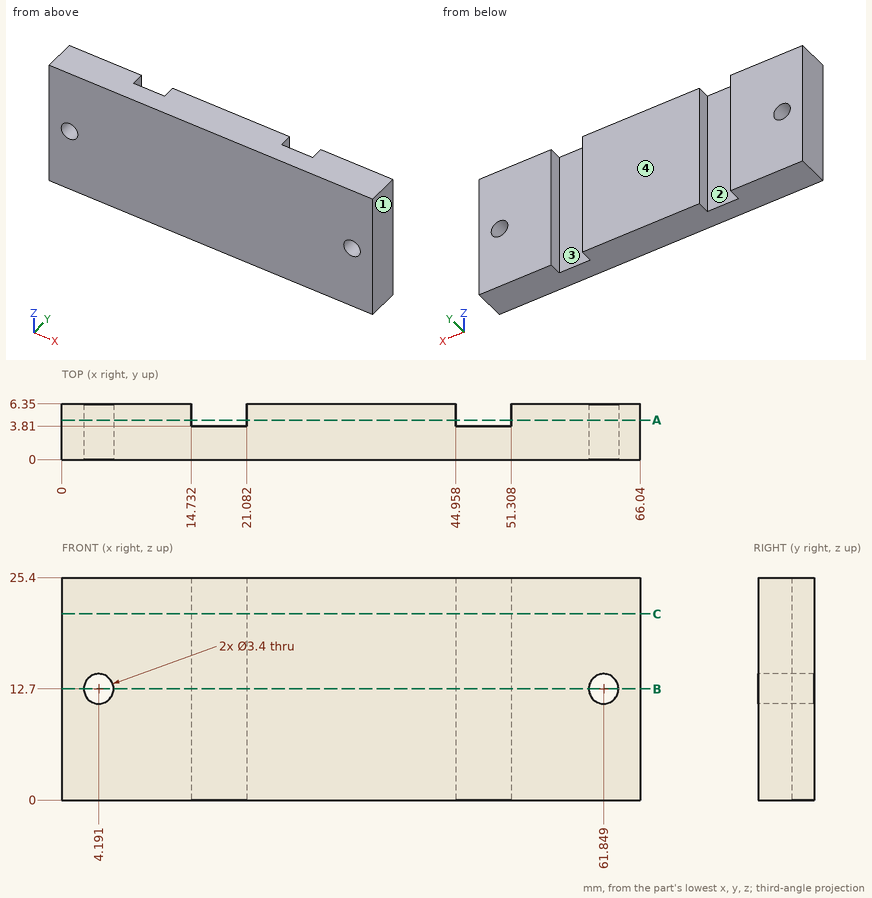
Input: dimensioned drawing with shaded views. Units: mm. Origin: part minimum x, y, z. Round coordinates to 2 decimals unless told otherwise and drop trailing zeros. Order: outer loops, then holes, each group sorted by start corner. A loop starts at its lowest first (then second) coordinate and runs counter-clockwise, first axis right, second up. Notation, with made-up numbers: (85.25, 78) - (128.25, 78) arc R7 ccw to (128.25, 87) - close; hole circle Ø2 at (18, 32). An arc over 180 degrees is marked (long way). Write item = value, one per line. Start each with the question number.
Q1. Cut plane A-A on y = 4.5. Return the cut outline in (x, z), and give its area (3 significant figures).
Q2. Ray query, line 1 (X direction, y = 5.75, z = 19); line 2 (X direction, y = 4.5, z = 12.7); line 3 (X direction, y = 3, z = 12.7). Return the intervals inside material, ascending. Write a range as from..to.
Q3. Cut plane C-C on z = 21.25. Return the cut outline in (x, y).
Q4. Cut plane B-B on z = 12.7. Return the cut outline in (x, y).
Q5. Pull-direction query (X, two-part tool) for the marked faces 1, 2, 3 and 4; classes: +X half, -X half, draft (parallel to the pull), parting line (faces both ways), or undercut.
Q6. Pin query (flat end, axial travel): pin 1 (1 mm diameter, centred on x = 46.5, y = 1, fed in from -Z); pin 2 (1.9 mm diameter, centred on x = 19, z = 9.5, fed in from +Y). Return the tip coordinate at first contact, or that it passes through.
Outcome:
q1.outline = (0, 0) - (14.73, 0) - (14.73, 25.4) - (0, 25.4) - close; (21.08, 0) - (44.96, 0) - (44.96, 25.4) - (21.08, 25.4) - close; (51.31, 0) - (66.04, 0) - (66.04, 25.4) - (51.31, 25.4) - close; hole circle Ø3.4 at (4.19, 12.7); hole circle Ø3.4 at (61.85, 12.7)
q1.area = 1,340 mm^2
q2.line_1 = 0..14.73, 21.08..44.96, 51.31..66.04
q2.line_2 = 0..2.49, 5.89..14.73, 21.08..44.96, 51.31..60.15, 63.55..66.04
q2.line_3 = 0..2.49, 5.89..60.15, 63.55..66.04
q3.outline = (0, 0) - (66.04, 0) - (66.04, 6.35) - (51.31, 6.35) - (51.31, 3.81) - (44.96, 3.81) - (44.96, 6.35) - (21.08, 6.35) - (21.08, 3.81) - (14.73, 3.81) - (14.73, 6.35) - (0, 6.35) - close
q4.outline = (0, 0) - (2.49, 0) - (2.49, 6.35) - (0, 6.35) - close; (5.89, 0) - (60.15, 0) - (60.15, 6.35) - (51.31, 6.35) - (51.31, 3.81) - (44.96, 3.81) - (44.96, 6.35) - (21.08, 6.35) - (21.08, 3.81) - (14.73, 3.81) - (14.73, 6.35) - (5.89, 6.35) - close; (63.55, 0) - (66.04, 0) - (66.04, 6.35) - (63.55, 6.35) - close
q5.face_1 = +X half
q5.face_2 = undercut
q5.face_3 = undercut
q5.face_4 = draft
q6.pin_1 = 0
q6.pin_2 = 3.81
